```python
from build123d import *

# Parameters (mm, degrees)
F0_W      = 38.1
F0_H      = 38.1
F1_DEPTH  = 38.1
F6_DEPTH  = 76.2
F8_DEPTH  = 76.2
F9_W      = 25.4
F9_H      = 7.62
F10_DEPTH = 76.2


with BuildPart() as f1:
    # F0 (on Front) → F1 (new body)
    with BuildSketch(Plane.XZ):
        with Locations((19.05, 19.05)):
            Rectangle(F0_W, F0_H)
    extrude(amount=F1_DEPTH)

    # F5 (on offset) → F6 (cut)
    with BuildSketch(Plane.YZ.offset(76.2)):
        Polygon((-11.43, 12.5278225169), (-6.35, 38.1), (-31.75, 38.1), (-26.67, 13.0124986172), (-21.59, 28.575), (-16.51, 28.575), align=None)
        Polygon((-25.4, 0), (-12.7, 0), (-19.05, 15.875), align=None)
        Polygon((-38.1, 0), (-31.75, 0), (-38.1, 38.1), align=None)
        Polygon((-6.35, 0), (0, 0), (0, 38.1), align=None)
    extrude(amount=-F6_DEPTH, mode=Mode.SUBTRACT)

    # F7 (on offset) → F8 (cut)
    with BuildSketch(Plane.XZ.offset(76.2)):
        Polygon((25.4, 38.1), (12.7, 38.1), (18.7603693128, 22.225), align=None)
        Polygon((6.35, 38.1), (0, 38.1), (0, 0), align=None)
        Polygon((11.43, 22.225), (6.35, 0), (31.75, 0), (26.67, 22.225), (21.59, 9.525), (16.51, 9.525), align=None)
        Polygon((38.1, 38.1), (31.75, 38.1), (38.1, 0), align=None)
    extrude(amount=-F8_DEPTH, mode=Mode.SUBTRACT)

    # F9 (on offset) → F10 (cut)
    with BuildSketch(Plane.XY.offset(76.2)):
        Polygon((38.1, -16.7285427451), (38.1, -9.1085427451), (12.7, -7.62), (12.7, -15.24), align=None)
        with Locations((12.7, -26.67)):
            Rectangle(F9_W, F9_H)
    extrude(amount=-F10_DEPTH, mode=Mode.SUBTRACT)


solid = f1.part
```
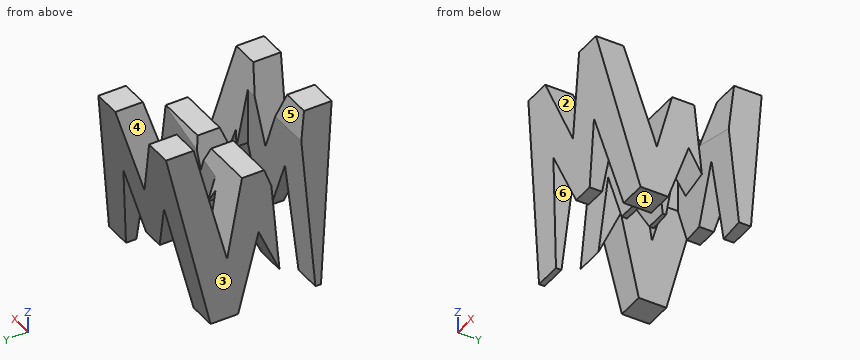
Could you check a few things on this model? Use its own coordinates, in mm. Face numbers are marked on the shaded views. A direction names the side the tool comes from. Coordinates: 2 decimals unless noted, no trailing zeros. Write each loop counter-clockwise with the first axis right and the second up, starting at its lowest first coordinate (ties: lowest second). Pieces come first, ordered by that corner, then holes. Notation, with made-up numbers: (62.25, -1.5) -> (97.25, -1.5) arc R21 ccw to (97.25, 33.5) -> close; hole circle Ø2 at (21, 27). An arc over 180 degrees is marked (long way). Write item = value, one per line. Start each with the question number.
(1) We'd pull the mould along X, two halves only. Please class the marked faces 1, 2 and 3: released by +X, released by -X, zero draft, split by the parting line, or undercut.
(2) Will these pins go through, and if not, where does the flat tip stop? pin 1 (8 mm diameter, centred on x = 23, z = 8, fed in from +Y); pin 2 (5.5 mm diameter, centred on x = 12.5, y = -20, fed in from +Z) (3 decimals); pin 3 (3 mm diameter, centred on y = -8.5, z = 26, fed in from +X); pin 4 (2 mm diameter, centred on x = 33.5, y = -28, fed in from -Z).
(3) I want a section at A-A (z = 4.5). Please give me the cut outline in (x, y), plus the area to 3 significant figures.
(4) I want a section at C-C (y = -34). Please give me the cut outline in (x, z) (3 decimals).
(5) Which directions (+Z, -Z, +X, -X, +Y, -Y) give clear straight access to the entire face, cutting with the end or side of a thin tool? Please do the marked faces 4, 5 and 6.
(6) I want a section at B-B (z = 23.5). Give the number of separate pieces and of enclosed holes in the cut face, plus the area to 3 significant figures.
(7) I need wall thicknesses on line 1 (Y direction, x = 21, z = 23); line 2 (Y direction, x = 29, z = 16); line 3 (X direction, y = -19, z = 21.5). Which ranges of each line are inside material? Lowest first, please. Write a range as [from, to].
Result set:
q1.face_1 = zero draft
q1.face_2 = undercut
q1.face_3 = released by -X
q2.pin_1 = -4.35
q2.pin_2 = 28.575
q2.pin_3 = 34.02
q2.pin_4 = 0
q3.outline = (0.75, -32.5) -> (7.38, -32.5) -> (7.38, -30.48) -> (0.75, -30.48) -> close; (0.75, -14.5) -> (7.38, -14.5) -> (7.38, -5.6) -> (0.75, -5.6) -> close; (30.72, -32.5) -> (37.35, -32.5) -> (37.35, -23.6) -> (30.72, -23.6) -> close; (30.72, -8.68) -> (37.35, -9.06) -> (37.35, -5.6) -> (30.72, -5.6) -> close
q3.area = 153 mm2
q4.outline = (2.25, 13.5) -> (9.436, 13.5) -> (11.43, 22.225) -> (14.92, 13.5) -> (23.18, 13.5) -> (26.67, 22.225) -> (28.664, 13.5) -> (35.85, 13.5) -> (31.75, 38.1) -> (25.4, 38.1) -> (18.76, 22.225) -> (12.7, 38.1) -> (6.35, 38.1) -> close
q5.face_4 = +Z, +Y, -Y
q5.face_5 = +Z, +X, -X
q5.face_6 = -Z, +Y, -Y
q6.separate_pieces = 6
q6.enclosed_holes = 0
q6.area = 562 mm2
q7.line_1 = [-35.58, -30.48], [-22.86, -15.73], [-8.11, -2.52]
q7.line_2 = [-34.42, -27.27], [-25.69, -16.2], [-8.58, -3.68]
q7.line_3 = [3.58, 11.26], [11.72, 26.38], [26.84, 34.52]
